Here's how the part is built. I have some questions about the finished solid (model axes, mm). Give positions to 0.01 mm unless a question says otherwise; leave off trailing zeros. Write each loop counter-clockwise with the first axis right and the second up, starting at its lowest first coordinate (ties: lowest second). Pieces come first, ordered by that corner, then holes. Notation, with made-up numbers: (-13, 44.25) - (38, 44.25) arc R29 cw to (38, 71.25) - close; hole circle Ø1 at (-12.75, 6). An arc over 180 degrees is marked (long way). Use one line per item in the form item = value. Start each with the question number.
from build123d import *

# Parameters (mm, degrees)
F0_R          = 8.875
F1_DEPTH      = 2
F1_DEPTH_BACK = 2
F2_SIZE       = 0.5
F3_T2_ANGLE   = 229.39221369
F3_T4_ANGLE   = 229.39221369
F3_T6_ANGLE   = 229.39221369
F3_T8_ANGLE   = 229.39221369


# Not quite as in the source:
# - a fillet or chamfer that OpenCascade refuses, or shapes differently, is made with other operations: its cross-section is extruded or revolved along the edge and cut away or added


with BuildPart() as f1:
    # F0 (on Front) → F1 (new body, two sides)
    with BuildSketch(Plane.XZ) as f1_sk:
        with BuildLine():
            ThreePointArc((9.0113523195, 6.7058048682), (5.1879898372, 10.5200364151), (0, 12.0204444975))
            ThreePointArc((0, 12.0204444975), (-5.1879898372, 10.5200364151), (-9.0113523195, 6.7058048682))
            ThreePointArc((-9.0113523195, 6.7058048682), (-9.186793263, -4.0631742687), (0, -9.6849640831))
            ThreePointArc((0, -9.6849640831), (9.186793263, -4.0631742687), (9.0113523195, 6.7058048682))
        make_face()
        Circle(F0_R, mode=Mode.SUBTRACT)
    extrude(amount=F1_DEPTH)
    extrude(f1_sk.sketch, amount=-F1_DEPTH_BACK)

    # F2
    f2_edges = [f1.edges().sort_by_distance(p)[0] for p in [
        (-8.875, 2, 0),
        (-8.875, -2, 0),
    ]]
    chamfer(f2_edges, length=F2_SIZE)

    # F3: fillet of radius 2 on 4 edges, made by hand

    # F3_s1 → F3_t2 (revolve, cut)
    with BuildSketch(Plane(origin=(-0.7137842207, 0, 0.3282453014), x_dir=(0, 1, 0), z_dir=(-0.9085365688, 0, 0.4178053412))):
        with BuildLine():
            ThreePointArc((2, 7.9336436901), (1.4142135624, 9.3478572525), (0, 9.9336436901))
            Line((0, 9.9336436901), (2, 9.9336436901))
            Line((2, 9.9336436901), (2, 7.9336436901))
        make_face()
    revolve(axis=Axis((-0.3277288129, 2, 1.1677402072), (0, -1, 0)), revolution_arc=F3_T2_ANGLE, mode=Mode.SUBTRACT)

    # F3_s3 → F3_t4 (revolve, cut)
    with BuildSketch(Plane(origin=(-0.1727441321, 0, 0.0794392031), x_dir=(0, 1, 0), z_dir=(0.9085365688, 0, -0.4178053412))):
        with BuildLine():
            ThreePointArc((2, 10.0555130523), (1.4142135624, 11.4697266146), (0, 12.0555130523))
            Line((0, 12.0555130523), (2, 12.0555130523))
            Line((2, 12.0555130523), (2, 10.0555130523))
        make_face()
    revolve(axis=Axis((0.3277288129, 2, 1.1677402072), (0, -1, 0)), revolution_arc=F3_T4_ANGLE, mode=Mode.SUBTRACT)

    # F3_s5 → F3_t6 (revolve, cut)
    with BuildSketch(Plane(origin=(0.1727441321, 0, 0.0794392031), x_dir=(0, 1, 0), z_dir=(-0.9085365688, 0, -0.4178053412))):
        with BuildLine():
            ThreePointArc((0, -12.0555130523), (-1.4142135624, -11.4697266146), (-2, -10.0555130523))
            Line((-2, -10.0555130523), (-2, -12.0555130523))
            Line((-2, -12.0555130523), (0, -12.0555130523))
        make_face()
    revolve(axis=Axis((-0.3277288129, -2, 1.1677402072), (0, 1, 0)), revolution_arc=F3_T6_ANGLE, mode=Mode.SUBTRACT)

    # F3_s7 → F3_t8 (revolve, cut)
    with BuildSketch(Plane(origin=(0.7137842207, 0, 0.3282453014), x_dir=(0, 1, 0), z_dir=(0.9085365688, 0, 0.4178053412))):
        with BuildLine():
            ThreePointArc((0, -9.9336436901), (-1.4142135624, -9.3478572525), (-2, -7.9336436901))
            Line((-2, -7.9336436901), (-2, -9.9336436901))
            Line((-2, -9.9336436901), (0, -9.9336436901))
        make_face()
    revolve(axis=Axis((0.3277288129, -2, 1.1677402072), (0, 1, 0)), revolution_arc=F3_T8_ANGLE, mode=Mode.SUBTRACT)


solid = f1.part
1. Please list where these lines run through material, in increasing order: line 1 (X direction, y = 1.35, z = 1); line 2 (Z direction, x = 0, y = -0.5) (3 decimals); line 3 (X direction, y = 0.6, z = 3.25).
2. For P1, Ø1.5, axis at x = 8, y = -0.5, coming from the -Z side, with a flat end and sliding along its axis, tell me the tip position at first contact or that it passes through.
3. We'd pull the mould along Z, two halves only. Please class faces 1 (the face through (0, 2, 9.6)), 2 (the face through (-1.173, -1.635, 8.934)), 3 (the face through (-1.173, 1.635, 8.934)): pulls with the +Z half, pulls with the -Z half, needs draft (parallel to the pull), parting line crosses it, or undercut.
4. I want a section at A-A, the plane y = -1.15. List the corners of the cut face in (x, z) for me (3 decimals), then the cut area to 3 significant figures.
5. I want a section at B-B, the plane y = 0.5. List the corners of the cut face in (x, z) for me (3 decimals).
Result sheet:
q1.line_1 = -10 to -8.82, 8.82 to 10
q1.line_2 = -9.621 to -8.875, 8.875 to 11.957
q1.line_3 = -10.23 to -8.26, 8.26 to 10.23
q2.P1 = -6.55
q3.face_1 = needs draft
q3.face_2 = undercut
q3.face_3 = undercut
q4.outline = (0, -9.321) arc R10.494 ccw to (0, 11.657) arc R10.494 ccw to start; hole circle Ø17.75 at (0, 0)
q4.area = 84.8 mm2
q5.outline = (0, -9.621) arc R10.794 ccw to (0, 11.957) arc R10.794 ccw to start; hole circle Ø17.75 at (0, 0)
